```python
from build123d import *

# Parameters (mm, degrees)
BOSS_EXTRUDE1_DEPTH = 10
CHAMFER1_SIZE       = 2


with BuildPart() as part:
    # Sketch1 → Boss-Extrude1 (new body)
    with BuildSketch(Plane(origin=(0, 0, 0), x_dir=(1, 0, 0), z_dir=(0, 1, 0))):
        Polygon((7.7, 26.75), (-7.7, 26.75), (-7.7, -26.75), (7.7, -26.75), (7.7, -31.75), (-12.7, -31.75), (-12.7, 31.75), (7.7, 31.75), align=None)
    extrude(amount=BOSS_EXTRUDE1_DEPTH)

    # Chamfer1
    chamfer1_edges = [part.edges().sort_by_distance(p)[0] for p in [
        (7.7, 5, -26.75),
        (-7.7, 5, -26.75),
        (-7.7, 5, 26.75),
        (7.7, 5, 26.75),
    ]]
    chamfer(chamfer1_edges, length=CHAMFER1_SIZE)


solid = part.part
```
Check sheet for the modelled part. Datum: model origin and axes. Units: mm. A direction names the side the tool comes from. Round coordinates to 2 decimals unless told otherwise and drop trailing zeros. Order: outer loops, then holes, each group sorted by start corner. A loop starts at its lowest first (then second) coordinate and runs counter-clockwise, first axis right, second up.
1) Section check C-C (z = 15). Record the boundary of the cut face in (x, y), and give its area (3 significant figures).
2) Scan lines: line 1 (Z direction, x = 2.75, y = 9.5); line 2 (X direction, y = 9.75, z = -18). Record each from-to range of solid material in increasing order.
3) Go/stop test with a flat-tipped pin: pin 1 Ø8 at (x, z) = (-3.5, 9.5) entering from -Y. Record where the tip stops, or that it passes through.
4) Section check A-A (x = 3.75). Record the boundary of the cut face in (y, z).
5) Mould release check, pull along Z, two halves, no side actions. Record for faces 1 (the flat face through (6.71, 4.93, -27.76)), 2 (the flat face through (0, 5, 26.75)), 3 (the flat face through (-2, 5, 31.75)), 4 (the flat face through (7.7, 5, -30)): +Z half, -Z half, draft (parallel to the pull), parting line (faces both ways), or undercut.
6) Section check B-B (y = 8.75). Record the boundary of the cut face in (x, z), and give its area (4 significant figures).
7) Section check D-D (x = -6.75). Record the boundary of the cut face in (y, z).
8) Tool access check on faces 5 (the flat face through (-7.7, 5, 0)), 6 (the flat face through (-3, 5, -31.75)). Record the directions out of +Z, -Z, +X, -X, +Y, -Y that give a thin tool (end or side, any length) a straight path to the whole face; none if there is none.
Result:
1. outline: (-12.7, 0) - (-7.7, 0) - (-7.7, 10) - (-12.7, 10) - close
1. area: 50.0 mm2
2. line 1: z = -31.75 to -26.75, 26.75 to 31.75
2. line 2: x = -12.7 to -7.7
3. pin 1: passes through
4. outline: (0, -31.75) - (10, -31.75) - (10, -26.75) - (0, -26.75) - close; (0, 26.75) - (10, 26.75) - (10, 31.75) - (0, 31.75) - close
5. face 1: undercut
5. face 2: undercut
5. face 3: +Z half
5. face 4: draft
6. outline: (-12.7, -31.75) - (7.7, -31.75) - (7.7, -28.75) - (5.7, -26.75) - (-5.7, -26.75) - (-7.7, -24.75) - (-7.7, 24.75) - (-5.7, 26.75) - (5.7, 26.75) - (7.7, 28.75) - (7.7, 31.75) - (-12.7, 31.75) - close
6. area: 471.5 mm2
7. outline: (0, -31.75) - (10, -31.75) - (10, -25.7) - (0, -25.7) - close; (0, 25.7) - (10, 25.7) - (10, 31.75) - (0, 31.75) - close
8. face 5: +X, +Y, -Y
8. face 6: -Z, +X, -X, +Y, -Y
